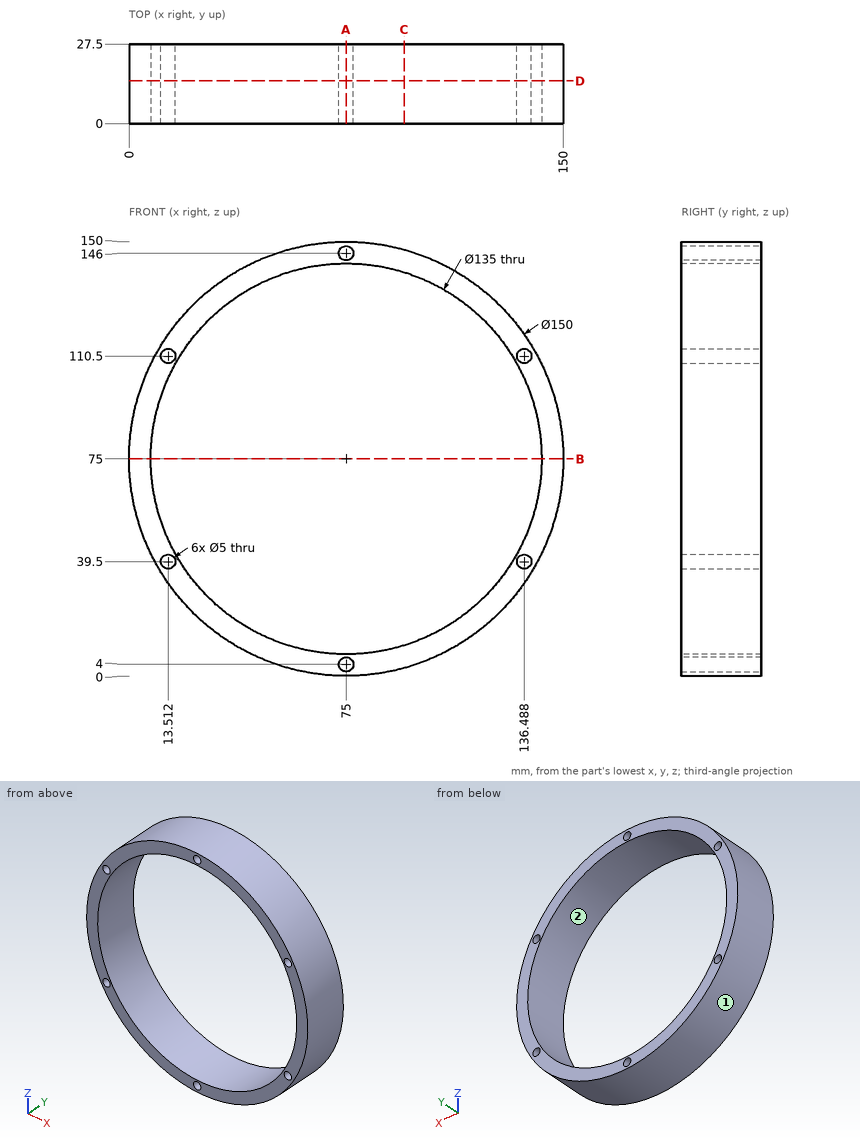
Geometry: see drawing. Coordinates: mm, zero at the bounding-box minimum. Give positions to 0.01 mm unless a question says otherwise; leave off trailing zeros. Loops run counter-clockwise (first coordinate to the right, second up) from the corner with the lowest first, then second, coordinate; pieces in that order, holes last. Notation, with made-up numbers: M -27.5,-30 L 0.5,-30 A20 cw 0.5,2 Z; hole C 78,-36.75 d6. An arc over 180 degrees is marked long. Answer as CSV lines item,"result". Start each with the question number.
1. Section B-B on z = 75. Return loops of the section in (x, y).
2. Section C-C on x = 95. Return loops of the section in (y, z).
3. Section A-A on x = 75. Return loops of the section in (y, z).
4. Pull-direction query (Z, two-part tool) for the marked faces 1 and 2; classes: released by +Z, released by -Z, zero draft, split by the parting line, or undercut.
5. Line query: L1, parallel to X at y = 18.5, z = 109; L2, parallel to X at y = 16.5, z = 110.5; L3, parallel to Z at x = 133, y = 22.75. Output: solid intervals per line, ascending.
6. Section D-D on y = 14.75. Return loops of the section in (x, z), plus the area to 3 significant figures.
7. Pin query (flat end, axial travel): P1, Ø3, axis at y = 19, z = 31, coming from the +X side; P2, Ø3, axis at x = 75, z = 4, coming from the -Y side; P3, Ø4, axis at x = 57, y = 13.5, coming from the -Z side; P4, Ø6, axis at y = 21, z = 40, coming from the +X side. Return the tip coordinate at first contact, or that it passes through.
Computed values:
1,outline,"M 0,0 L 7.5,0 L 7.5,27.5 L 0,27.5 Z; M 142.5,0 L 150,0 L 150,27.5 L 142.5,27.5 Z"
2,outline,"M 0,2.72 L 27.5,2.72 L 27.5,10.53 L 0,10.53 Z; M 0,139.47 L 27.5,139.47 L 27.5,147.28 L 0,147.28 Z"
3,outline,"M 0,0 L 27.5,0 L 27.5,1.5 L 0,1.5 Z; M 0,6.5 L 27.5,6.5 L 27.5,7.5 L 0,7.5 Z; M 0,142.5 L 27.5,142.5 L 27.5,143.5 L 0,143.5 Z; M 0,148.5 L 27.5,148.5 L 27.5,150 L 0,150 Z"
4,face 1,"split by the parting line"
4,face 2,"undercut"
5,L1,"x = 8.15 to 11.51, 15.51 to 16.69, 133.31 to 134.49, 138.49 to 141.85"
5,L2,"x = 8.93 to 11.01, 16.01 to 17.59, 132.41 to 133.99, 138.99 to 141.07"
5,L3,"z = 27.45 to 40.47, 109.53 to 122.55"
6,outline,"C 75,75 d150; hole C 75,75 d135; hole C 13.51,39.5 d5; hole C 13.51,110.5 d5; hole C 75,4 d5; hole C 75,146 d5; hole C 136.49,39.5 d5; hole C 136.49,110.5 d5"
6,area,"3,240 mm²"
7,P1,"stops at x = 136.8"
7,P2,"passes through"
7,P3,"stops at z = 1.73"
7,P4,"stops at x = 142.83"
